Autodesk Inventor part; units mm, degrees
ref_plane "YZ Plane" through (0, 0, 0) normal (1, 0, 0) x (0, 1, 0)
ref_plane "XZ Plane" through (0, 0, 0) normal (0, 1, 0) x (-1, 0, 0)
ref_plane "XY Plane" through (0, 0, 0) normal (0, 0, 1) x (1, 0, 0)
sketch "Sketch1" plane through (0, 0, 0) normal (0, 0, 1) x (1, 0, 0)
  line L0 (-27.669, 1.4923) -> (-27.669, 15.9923)
  line L1 (-27.669, 15.9923) -> (-47.669, 15.9923)
  line L2 (-47.669, 15.9923) -> (-47.669, 1.4923)
  line L3 (4.7848, 57.9257) -> (-7.7725, 50.6757)
  line L4 (-7.7725, 50.6757) -> (-17.7732, 67.9973)
  line L5 (-17.7732, 67.9973) -> (-5.2158, 75.2473)
  circle A0 centre (-1.2464, 23.3799) radius 2.05
  line L6 (-47.669, 1.4923) -> (-67.669, 1.4923)
  line L7 (-27.669, 1.4923) -> (-0.5414, 1.7834)
  line L8 (4.7848, 57.9257) -> (18.3286, 34.4672)
  line L9 (-0.7095, 1.4923) -> (18.3286, 34.4672)
  line L10 (-15.2158, 92.5678) -> (-5.2158, 75.2473)
  line L11 (-47.669, 1.4923) -> (-67.669, 1.4923)
  line L12 (-67.669, 1.4923) -> (-67.669, 11.5002)
  line L13 (-47.669, 11.5) -> (-47.669, 1.4923)
  line L14 (-5.2158, 75.2473) -> (-15.2158, 92.5678)
  line L15 (-15.2158, 92.5678) -> (-23.5411, 87.7613)
  line L16 (-13.8463, 70.2645) -> (-5.2158, 75.2473)
  line L17 (-5.2158, 75.2473) -> (14.7842, 75.2473) construction
  line L18 (-23.5411, 87.7613) -> (-67.669, 11.5002)
  line L19 (18.3286, 34.4672) -> (22.6587, 36.9672)
  line L20 (-0.7095, 1.4923) -> (-0.7095, -3.5077)
  line L21 (-67.669, 1.4923) -> (-67.669, -3.5077)
  line L22 (-47.669, 1.4923) -> (-47.669, -3.5077)
  line L23 (-47.669, -3.5077) -> (-67.669, -3.5077)
  line L24 (-27.669, 1.4923) -> (-27.669, -3.5077)
  line L25 (-27.669, -3.5077) -> (-0.7095, -3.5077)
  line L26 (4.7848, 57.9257) -> (9.115, 60.4257)
  line L27 (9.115, 60.4257) -> (22.6587, 36.9672)
  line L28 (-15.2158, 92.5678) -> (-10.8857, 95.0678)
  line L29 (-5.2158, 75.2473) -> (-0.8857, 77.7473)
  line L30 (-0.8857, 77.7473) -> (-10.8857, 95.0678)
  line L31 (-23.5411, 87.7613) -> (-18.5411, 87.7613) construction
  line L32 (-0.7095, 1.4923) -> (3.6206, -1.0077)
  line L33 (-0.7095, 1.4923) -> (4.2905, 1.4923) construction
  line L34 (18.3286, 34.4672) -> (22.6587, 31.9672)
  line L35 (18.3286, 34.4672) -> (23.3286, 34.4672) construction
  line L36 (-67.669, 11.5002) -> (-71.9991, 14.0002)
  line L37 (-67.669, 11.5002) -> (-62.669, 11.5002) construction
  line L38 (-23.5411, 87.7613) -> (-27.8713, 90.261)
  line L39 (-27.8713, 90.261) -> (-71.9991, 14.0002)
  line L40 (3.6206, -1.0077) -> (22.6587, 31.9672)
  line L41 (-71.9991, 14.0002) -> (-71.9991, -3.5077)
  line L42 (-71.9991, -3.5077) -> (-67.669, -3.5077)
  line L43 (-10.8857, 95.0678) -> (-13.0507, 98.8177)
  line L44 (-13.0507, 98.8177) -> (-27.8713, 90.261)
  line L45 (22.6587, 31.9672) -> (22.6587, 36.9672)
  line L46 (-0.7095, -3.5077) -> (3.6206, -1.0077)
  point P0 (0, 0)
  point P1 (0, 0)
  dimension "d19" = 4.1
  dimension "d21" = 20
  dimension "d23" = 20
  dimension "d24" = 120
  dimension "d26" = 5
  dimension "d27" = 5
  dimension "d28" = 5
  dimension "d29" = 5
  dimension "d30" = 5
  dimension "d31" = 5
  dimension "d32" = 5
  dimension "d33" = 5
  dimension "d39" = 5
  dimension "d40" = 30
  dimension "d41" = 5
  dimension "d42" = 30
  dimension "d43" = 5
  dimension "d44" = 150
  dimension "d45" = 5
  dimension "d46" = 4.33
  dimension "d55" = 90
  dimension "d56" = 120
  dimension "d57" = 90
  dimension "d58" = 90
extrude "Extrusion1" add sketch "Sketch1" along normal blind 20
sketch "Sketch4" plane through (-27.669, -3.5077, 0) normal (-1, 0, 0) x (0, 0, 1)
  line L0 (20, 19.5) -> (20, 0)
  line L1 (0, 19.5) -> (20, 19.5)
  line L2 (20, 0) -> (18, 0)
  line L3 (18, 0) -> (18, 19.5)
  line L4 (18, 19.5) -> (20, 19.5)
  line L5 (20, 19.5) -> (20, 0)
  point P0 (0, 3.5077)
  dimension "d59" = 2
extrude "Extrusion4" add sketch "Sketch4" along normal blind 20
sketch "Sketch5" plane through (-0.8857, 77.7473, 0) normal (0.5, -0.8660254, 0) x (0.8660254, 0.5, 0)
  line L0 (0, 0) -> (0, 20)
  line L1 (0, 20) -> (-19.5, 20)
  line L2 (-19.5, 20) -> (-19.5, 18)
  line L3 (-19.5, 18) -> (0, 18)
  line L4 (0, 18) -> (0, 20)
  point P0 (-38.1066, 0)
  dimension "d62" = 19.5
  dimension "d63" = 2
extrude "Extrusion5" add sketch "Sketch5" along normal blind 21
sketch "Sketch7" plane through (0, 0, 0) normal (0, 0, -1) x (-1, 0, 0)
  line L0 (0, 0) -> (0, 23.3799)
  circle A0 centre (1.2464, 23.3799) radius 2.05
  line L1 (0, 23.3799) -> (1.2464, 23.3799)
hole "Hole1" at (-1.2464, 23.3799, 0) direction (0, 0, 1) diameter 5 end through all counterbore diameter 8.2 counterbore depth 10
sketch "Sketch8" plane through (-0.8857, 77.7473, 18) normal (0, 0, -1) x (-0.8660254, -0.5, 0)
  line L0 (0, 0) -> (0, -20.0013)
  line L1 (19.5, -20.0013) -> (0, -20.0013)
  line L2 (0, 0) -> (19.5, 0)
  line L3 (19.5, 0) -> (19.5, -20.0013)
  line L4 (19.5, -20.0013) -> (0, -20.0013)
  line L5 (0, -20.0013) -> (0, 0)
  point P0 (38.1066, -67.774)
extrude "Extrusion6" add sketch "Sketch8" along normal blind 8 and the other way blind 4
sketch "Sketch9" plane through (-27.669, -3.5077, 18) normal (0, 0, -1) x (-1, 0, 0)
  line L0 (20, 0) -> (20, 19.5)
  line L1 (0, 0) -> (20, 0)
  line L2 (20, 0) -> (20, 19.5)
  line L3 (20, 19.5) -> (0, 19.5)
  line L4 (0, 19.5) -> (0, 0)
  point P0 (-27.669, 3.5077)
extrude "Extrusion7" add sketch "Sketch9" along normal blind 8 and the other way blind 4
sketch "Sketch10" plane through (-0.8857, 77.7473, 22) normal (0, 0, 1) x (0.8660254, 0.5, 0)
  line L0 (0, 0) -> (-19.5, 0)
  line L1 (-19.5, -20.0013) -> (0, -20.0013)
  line L2 (0, 0) -> (-5, 0)
  line L3 (-5, 0) -> (-5, -20.0013)
  line L4 (-5, -20.0013) -> (0, -20.0013)
  line L5 (0, -20.0013) -> (0, 0)
  line L6 (-5, -20.0013) -> (-13.5, -20.0013)
  line L7 (-13.5, -20.0013) -> (-13.5, -10.0013)
  line L8 (-13.5, -10.0013) -> (-5, -10.0013)
  line L9 (-5, -10.0013) -> (-5, -20.0013)
  point P0 (-38.1066, -67.774)
  dimension "d81" = 5
  dimension "d82" = 8.5
  dimension "d83" = 10
hole "Hole2" at (-7.5764, 62.3359, 22) direction (0, 0, -1) diameter 4 end through all
sketch "Sketch11" plane through (-27.669, -3.5077, 22) normal (0, 0, 1) x (1, 0, 0)
  line L0 (-20, 0) -> (0, 0)
  line L1 (0, 0) -> (-20, 0)
  line L2 (-20, 0) -> (-20, 5)
  line L3 (-20, 5) -> (0, 5)
  line L4 (0, 5) -> (0, 0)
  line L5 (-20, 5) -> (-10, 5)
  line L6 (-10, 5) -> (-10, 13.5)
  line L7 (-10, 13.5) -> (-20, 13.5)
  line L8 (-20, 13.5) -> (-20, 5)
  point P0 (27.669, 3.5077)
  dimension "d91" = 20
  dimension "d92" = 5
  dimension "d93" = 10
  dimension "d101" = 8.5
hole "Hole3" at (-37.669, 9.9923, 22) direction (0, 0, -1) diameter 4 end through all
sketch "Sketch12" plane through (9.115, 60.4257, 20) normal (0.5, -0.8660254, 0) x (0.8660254, 0.5, 0)
  line L0 (0, 0) -> (-19.5, 0)
  line L1 (-19.5, 0) -> (-19.5, 2)
  line L2 (-19.5, 2) -> (0, 2)
  line L3 (0, 2) -> (0, 0)
  point P0 (-38.1066, -20)
extrude "Extrusion8" cut sketch "Sketch12" against normal blind 0.4
sketch "Sketch13" plane through (-17.7732, 67.9973, 22) normal (-0.5, 0.8660254, 0) x (0.8660254, 0.5, 0)
  line L0 (19.5, 0) -> (0, 0)
  line L1 (19.5, 2) -> (19.5, 0)
  line L2 (0, 0) -> (19.5, 0)
  line L3 (19.5, 0) -> (19.5, 2)
  line L4 (19.5, 2) -> (0, 2)
  line L5 (0, 2) -> (0, 0)
  point P0 (-18.6066, 22)
extrude "Extrusion9" cut sketch "Sketch13" against normal blind 0.4
sketch "Sketch14" plane through (-7.9725, 51.0221, 20) normal (-0.8660254, -0.5, 0) x (0, 0, 1)
  line L0 (0, 0) -> (0, 19.2013)
  line L1 (2, 19.2013) -> (2, 0)
  line L2 (0, 0) -> (2, 0)
  line L3 (2, 0) -> (2, 19.2013)
  line L4 (2, 19.2013) -> (0, 19.2013)
  line L5 (0, 19.2013) -> (0, 0)
  point P0 (-20, -48.1727)
extrude "Extrusion10" cut sketch "Sketch14" against normal blind 0.4
sketch "Sketch15" plane through (-47.669, -3.5077, 20) normal (-1, 0, 0) x (0, 0, 1)
  line L0 (0, 0) -> (2, 0)
  line L1 (2, 0) -> (2, 19.5)
  line L2 (2, 19.5) -> (0, 19.5)
  line L3 (0, 19.5) -> (0, 0)
  point P0 (-20, 3.5077)
extrude "Extrusion11" cut sketch "Sketch15" against normal blind 0.4
sketch "Sketch16" plane through (-27.669, -3.5077, 20) normal (1, 0, 0) x (0, 0, -1)
  line L0 (0, 19.5) -> (0, 0)
  line L1 (-2, 0) -> (-2, 19.5)
  line L2 (0, 0) -> (-2, 0)
  line L3 (-2, 0) -> (-2, 19.5)
  line L4 (-2, 19.5) -> (0, 19.5)
  line L5 (0, 19.5) -> (0, 0)
  point P0 (20, 3.5077)
extrude "Extrusion12" cut sketch "Sketch16" against normal blind 0.4
sketch "Sketch17" plane through (-47.269, 15.9923, 22) normal (0, 1, 0) x (1, 0, 0)
  line L0 (19.2, 0) -> (0, 0)
  line L1 (0, 2) -> (19.2, 2)
  line L2 (19.2, 2) -> (19.2, 0)
  line L3 (19.2, 0) -> (0, 0)
  line L4 (0, 0) -> (0, 2)
  point P0 (47.269, 22)
extrude "Extrusion13" cut sketch "Sketch17" against normal blind 0.4
properties part number "Delta Feet"
Design review of the part built by this model. Coordinates are the model's own, in mm. A direction names the side the tool comes from. Round coordinates to 2 decimals unless told otherwise and drop trailing zeros. Order: outer loops, then holes, each group sorted by start corner. A loop starts at its lowest first (then second) coordinate and runs counter-clockwise, first axis right, second up. Notation, with made-up numbers: M 50.5,57.25 L 70.5,57.25 A33 ccw 70.5,95.25 Z; hole C -31,-19.5 d10. An arc over 180 degrees is marked long. Put each result on its own line as item: value.
Q1. To check wall thickness, follow line 1 (Z direction, x = -52.5, y = 30.5); line 2 (X direction, y = 25, z = 18.5); line 3 (X direction, y = 2, z = 6.5). State the ranges of each line that lie inside material, in increasing order.
Reported:
line 1: 0 to 20
line 2: -65.63 to -3.15, 0.66 to 18.64
line 3: -72 to -47.67, -27.67 to 5.36
Q2. Consider section B-B (z = 7.75). State the section outline as (x, y) points (1 decimal), and give its area (3 significant figures).
Reported:
outline: M -72,-3.5 L -47.7,-3.5 L -47.7,16 L -27.7,16 L -27.7,-3.5 L -0.7,-3.5 L 3.6,-1 L 22.7,32 L 22.7,37 L 9.1,60.4 L 4.8,57.9 L -7.8,50.7 L -17.8,68 L -5.2,75.2 L -0.9,77.7 L -10.9,95.1 L -13.1,98.8 L -27.9,90.3 L -72,14 Z; hole C -1.2,23.4 d8.2
area: 5,260 mm²
Q3. Consider section C-C (x = -45). State the section outline as (y, z) points.
Reported:
outline: M -3.51,10 L 15.99,10 L 15.99,0 L 60.66,0 L 60.66,20 L 15.59,20 L 15.59,22 L -3.51,22 Z
Q4. Draft analysis for pull direction X (two halves, no side actions). For faces 1 (the face through (-12.49, 59.65, 20.99)), 2 (the face through (-4, 64, 10)), 3 (the face through (-25, 37, 0)), 4 (the face through (22.659, 34, 10)), state which applies: released by +X, released by -X, zero draft, split by the parting line, or undercut.
Reported:
face 1: released by -X
face 2: undercut
face 3: zero draft
face 4: released by +X
Q5. Machinability: for faces 5 (the face through (-27.669, 6, 5)), 6 (the face through (-38, 6, 22)), 7 (the face through (-12.703, 59.215, 4.93)), which of the approach directions +Z, -Z, +X, -X, +Y, -Y give a long, thin tool a straight path to every point of the face, cutting with its end or side? Answer none if there is none.
Reported:
face 5: -Z, -Y
face 6: +Z, +X, -X, +Y, -Y
face 7: -Z
Q6. Insertion check: pin 1 Ø0.6 at (y, z) = (6, 20.5) entering from -X; pin 2 Ø5 at (x, z) = (-0.5, 14.5) entering from +Y; pin 3 Ø4 at (x, z) = (-40.5, 18.5) entering from +Y. Each pin has a flat end and moves straight along its axis. Give the tip position at first contact, or say it passes through.
Reported:
pin 1: x = -47.27
pin 2: y = 81.41
pin 3: y = 71.89
Q7. Consider section A-A (x = -2.5). State the section outline as (y, z) points.
Reported:
outline: M -3.51,0 L 19.48,0 L 19.48,10 L 21.22,10 L 21.22,20 L -3.51,20 Z; M 25.54,10 L 27.28,10 L 27.28,0 L 53.72,0 L 53.72,10 L 76.82,10 L 76.82,0 L 80.54,0 L 80.54,20 L 76.35,20 L 76.35,22 L 54.18,22 L 54.18,20 L 25.54,20 Z
Q8. Consider section D-D (y = 46.5). State the section outline as (x, z) points.
Reported:
outline: M -53.19,0 L 17.15,0 L 17.15,20 L -53.19,20 Z
